Here's how the part is built. I have some questions about the finished solid (model axes, mm). Face numbers are marked on the shaded views. A direction names the side the tool comes from. Give positions to 0.01 mm unless a question says otherwise; leave off trailing zeros. Write each loop counter-clockwise with the first axis right and the second up, starting at its lowest first coordinate (ties: lowest second). Pieces come first, ordered by that corner, then holes. Notation, with made-up numbers: (3, 59.25) - (22, 59.25) arc R11 ccw to (22, 80.25) - close; hole circle Ø8 at (31.5, -2.75). An arc over 180 degrees is marked (long way). Use a Markdown table: item, result.
```python
from build123d import *

# Parameters (mm, degrees)
SKETCH_W        = 35
SKETCH_H        = 13.6
PAD_DEPTH       = 12.5
SKETCH001_R     = 6
POCKET_DEPTH    = 13.601
SKETCH002_R     = 2
POCKET001_DEPTH = 12.501
SKETCH003_R     = 8
POCKET002_DEPTH = 4
SKETCH004_R     = 8
POCKET003_DEPTH = 4


with BuildPart() as part:
    # Sketch → Pad (new body)
    with BuildSketch(Plane.XY):
        Rectangle(SKETCH_W, SKETCH_H)
    extrude(amount=PAD_DEPTH)

    # Sketch001 (on Face3 of Pad) → Pocket (cut, through all)
    with BuildSketch(Plane.XZ.offset(6.8)):
        with Locations((0, 12.5)):
            Circle(SKETCH001_R)
    extrude(amount=-POCKET_DEPTH, mode=Mode.SUBTRACT)

    # Sketch002 (on Face2 of Pocket) → Pocket001 (cut, through all)
    with BuildSketch(Plane(origin=(0, 0, 0), x_dir=(1, 0, 0), z_dir=(0, 0, -1))):
        with Locations((-12.5, 0)):
            Circle(SKETCH002_R)
        with Locations((12.5, 0)):
            Circle(SKETCH002_R)
    extrude(amount=-POCKET001_DEPTH, mode=Mode.SUBTRACT)

    # Sketch003 (on Face8 of Pocket001) → Pocket002 (cut)
    with BuildSketch(Plane.XZ.offset(6.8)):
        with Locations((0, 12.5)):
            Circle(SKETCH003_R)
    extrude(amount=-POCKET002_DEPTH, mode=Mode.SUBTRACT)

    # Sketch004 (on Face1 of Pocket002) → Pocket003 (cut)
    with BuildSketch(Plane(origin=(0, 6.8, 0), x_dir=(-1, 0, 0), z_dir=(0, 1, 0))):
        with Locations((0, 12.5)):
            Circle(SKETCH004_R)
    extrude(amount=-POCKET003_DEPTH, mode=Mode.SUBTRACT)


solid = part.part
```
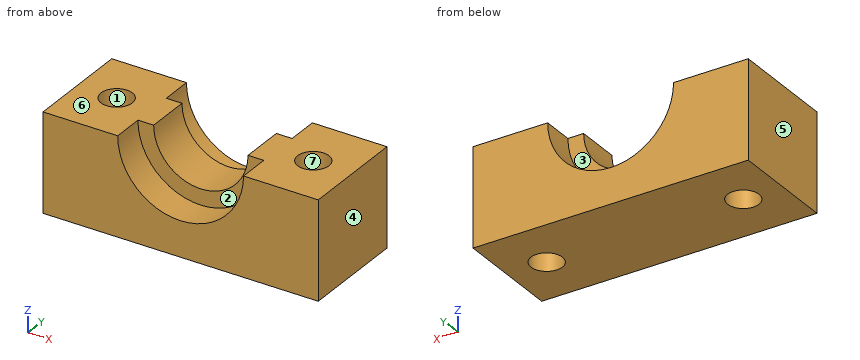
Item 1: If we section it at D-D, the plane z = 4: Write out the boundary of the cut face in (x, y), plus the area to 3 significant figures.
Values:
| item | result |
|---|---|
| outline | (-17.5, -6.8) - (17.5, -6.8) - (17.5, 6.8) - (-17.5, 6.8) - close; hole circle Ø4 at (-12.5, 0); hole circle Ø4 at (12.5, 0) |
| area | 451 mm2 |
Item 2: I need wall thicknesses on line 1 along X through (y, z) = (0, 3); line 2 along Y through (x, z) = (12.5, 10); line 3 along X through (y, z) = (0, 7.5). Which ranges of each line are inside material? Lowest first, please. Write a range as [from, to].
Values:
| item | result |
|---|---|
| line 1 | x = [-17.5, -14.5], [-10.5, 10.5], [14.5, 17.5] |
| line 2 | y = [-6.8, -2], [2, 6.8] |
| line 3 | x = [-17.5, -14.5], [-10.5, -3.32], [3.32, 10.5], [14.5, 17.5] |
Item 3: If we section it at C-C, the plane x = 13.5: Write out the boundary of the cut face in (y, z), plus the area to 3 significant figures.
Values:
| item | result |
|---|---|
| outline | (-6.8, 0) - (-1.73, 0) - (-1.73, 12.5) - (-6.8, 12.5) - close; (1.73, 0) - (6.8, 0) - (6.8, 12.5) - (1.73, 12.5) - close |
| area | 127 mm2 |
Item 4: If we section it at B-B, the plane z = 11.5: Write out the boundary of the cut face in (x, y), plus the area to 3 significant figures.
Values:
| item | result |
|---|---|
| outline | (-17.5, -6.8) - (-7.94, -6.8) - (-7.94, -2.8) - (-5.92, -2.8) - (-5.92, 2.8) - (-7.94, 2.8) - (-7.94, 6.8) - (-17.5, 6.8) - close; (5.92, -2.8) - (7.94, -2.8) - (7.94, -6.8) - (17.5, -6.8) - (17.5, 6.8) - (7.94, 6.8) - (7.94, 2.8) - (5.92, 2.8) - close; hole circle Ø4 at (-12.5, 0); hole circle Ø4 at (12.5, 0) |
| area | 258 mm2 |
Item 5: Thinking about a two-plate mould opening in X: for the marked faces 4, 5, 6 and 7, which applies, +X half, -X half, draft (parallel to the pull), parting line (faces both ways), or undercut?
Values:
| item | result |
|---|---|
| face 4 | +X half |
| face 5 | -X half |
| face 6 | draft |
| face 7 | undercut |
Item 6: If we section it at A-A, the plane y = 0: Write out the boundary of the cut face in (x, z), plus the area to 3 significant figures.
Values:
| item | result |
|---|---|
| outline | (-17.5, 0) - (-14.5, 0) - (-14.5, 12.5) - (-17.5, 12.5) - close; (-10.5, 0) - (10.5, 0) - (10.5, 12.5) - (6, 12.5) arc R6 cw to (-6, 12.5) - (-10.5, 12.5) - close; (14.5, 0) - (17.5, 0) - (17.5, 12.5) - (14.5, 12.5) - close |
| area | 281 mm2 |
Item 7: For the marked faces 1, 2 and 3, which set-ups out of +Z, -Z, +X, -X, +Y, -Y let a thin tool reach every point of the face, with its end or its side?
Values:
| item | result |
|---|---|
| face 1 | +Z, -Z |
| face 2 | +Z, -Y |
| face 3 | +Z, +Y |
Item 8: Will this pin go through, and if not, where does the flat tip stop? pin 1 Ø1 at (x, y) = (-9, 4.5) entering from -Z.
Values:
| item | result |
|---|---|
| pin 1 | stops at z = 0 |
